from build123d import *

# Parameters (mm, degrees)
SKETCH1_W                    = 94
SKETCH1_H                    = 75
BASE_FLANGE1_DEPTH           = 1.5
EDGE_FLANGE1_DEPTH           = 75
EDGE_FLANGE2_STRIP_W         = 16
EDGE_FLANGE2_STRIP_H         = 1.5
EDGE_FLANGE2_STRIP_CUT_DEPTH = 75
EDGE_FLANGE2_DEPTH           = 75
EDGE_FLANGE3_DEPTH           = 75
EDGE_FLANGE4_STRIP_W         = 16
EDGE_FLANGE4_STRIP_H         = 1.5
EDGE_FLANGE4_STRIP_CUT_DEPTH = 75
EDGE_FLANGE4_DEPTH           = 75
SKETCH18_R                   = 7.5
CUT_EXTRUDE1_DEPTH           = 10
EDGE_FLANGE5_DEPTH           = 94
EDGE_FLANGE6_DEPTH           = 94


# Sheet-metal steps are written as plain solids
with BuildPart() as part:
    # Sketch1 → Base-Flange1 (new body)
    with BuildSketch(Plane.XY):
        Rectangle(SKETCH1_W, SKETCH1_H)
        with BuildLine():
            Line((5, 25.5), (5, 13.5))
            ThreePointArc((5, 13.5), (0, 8.5), (-5, 13.5))
            Line((-5, 13.5), (-5, 25.5))
            ThreePointArc((-5, 25.5), (0, 30.5), (5, 25.5))
        make_face(mode=Mode.SUBTRACT)
        with BuildLine():
            Line((19.583647797, -17.080127019), (9.191342951, -11.080127019))
            ThreePointArc((9.191342951, -11.080127019), (7.361215932, -4.25), (14.191342951, -2.419872981))
            Line((14.191342951, -2.419872981), (24.583647797, -8.419872981))
            ThreePointArc((24.583647797, -8.419872981), (26.413774815, -15.25), (19.583647797, -17.080127019))
        make_face(mode=Mode.SUBTRACT)
        with BuildLine():
            Line((-24.583647797, -8.419872981), (-14.191342951, -2.419872981))
            ThreePointArc((-14.191342951, -2.419872981), (-7.361215932, -4.25), (-9.191342951, -11.080127019))
            Line((-9.191342951, -11.080127019), (-19.583647797, -17.080127019))
            ThreePointArc((-19.583647797, -17.080127019), (-26.413774815, -15.25), (-24.583647797, -8.419872981))
        make_face(mode=Mode.SUBTRACT)
    extrude(amount=-BASE_FLANGE1_DEPTH)

    # Edge-Flange1 section (across the edge) → Edge-Flange1 (add)
    with BuildSketch(Plane(origin=(49, -37.5, 0), x_dir=(-1, 0, 0), z_dir=(0, 1, 0))):
        with BuildLine():
            Line((-1.5, 2), (-1.5, 18.5))
            Line((-1.5, 18.5), (0, 18.5))
            Line((0, 18.5), (0, 2))
            ThreePointArc((0, 2), (0.585786438, 0.585786438), (2, 0))
            Line((2, 0), (2, -1.5))
            ThreePointArc((2, -1.5), (-0.474873734, -0.474873734), (-1.5, 2))
        make_face()
    extrude(amount=EDGE_FLANGE1_DEPTH)

    # Edge-Flange2 strip (across the edge) → Edge-Flange2 strip cut (cut)
    with BuildSketch(Plane(origin=(50.5, 37.5, 18.5), x_dir=(0, 0, -1), z_dir=(0, -1, 0))):
        with Locations((-3, -0.75)):
            Rectangle(EDGE_FLANGE2_STRIP_W, EDGE_FLANGE2_STRIP_H)
    extrude(amount=EDGE_FLANGE2_STRIP_CUT_DEPTH, mode=Mode.SUBTRACT)

    # Edge-Flange2 section (across the edge) → Edge-Flange2 (add)
    with BuildSketch(Plane(origin=(50.5, 37.5, 18.5), x_dir=(0, 0, -1), z_dir=(0, -1, 0))):
        with BuildLine():
            Line((-1.5, 5), (-1.5, 48.5))
            Line((-1.5, 48.5), (0, 48.5))
            Line((0, 48.5), (0, 5))
            ThreePointArc((0, 5), (1.464466094, 1.464466094), (5, 0))
            Line((5, 0), (5, -1.5))
            ThreePointArc((5, -1.5), (0.403805922, 0.403805922), (-1.5, 5))
        make_face()
    extrude(amount=EDGE_FLANGE2_DEPTH)

    # Edge-Flange3 section (across the edge) → Edge-Flange3 (add)
    with BuildSketch(Plane(origin=(-49, 37.5, 0), x_dir=(1, 0, 0), z_dir=(0, -1, 0))):
        with BuildLine():
            Line((-1.5, 2), (-1.5, 18.5))
            Line((-1.5, 18.5), (0, 18.5))
            Line((0, 18.5), (0, 2))
            ThreePointArc((0, 2), (0.585786438, 0.585786438), (2, 0))
            Line((2, 0), (2, -1.5))
            ThreePointArc((2, -1.5), (-0.474873734, -0.474873734), (-1.5, 2))
        make_face()
    extrude(amount=EDGE_FLANGE3_DEPTH)

    # Edge-Flange4 strip (across the edge) → Edge-Flange4 strip cut (cut)
    with BuildSketch(Plane(origin=(-50.5, -37.5, 18.5), x_dir=(0, 0, -1), z_dir=(0, 1, 0))):
        with Locations((-3, -0.75)):
            Rectangle(EDGE_FLANGE4_STRIP_W, EDGE_FLANGE4_STRIP_H)
    extrude(amount=EDGE_FLANGE4_STRIP_CUT_DEPTH, mode=Mode.SUBTRACT)

    # Edge-Flange4 section (across the edge) → Edge-Flange4 (add)
    with BuildSketch(Plane(origin=(-50.5, -37.5, 18.5), x_dir=(0, 0, -1), z_dir=(0, 1, 0))):
        with BuildLine():
            Line((-1.5, 5), (-1.5, 48.5))
            Line((-1.5, 48.5), (0, 48.5))
            Line((0, 48.5), (0, 5))
            ThreePointArc((0, 5), (1.464466094, 1.464466094), (5, 0))
            Line((5, 0), (5, -1.5))
            ThreePointArc((5, -1.5), (0.403805922, 0.403805922), (-1.5, 5))
        make_face()
    extrude(amount=EDGE_FLANGE4_DEPTH)

    # Sketch18 → Cut-Extrude1 (cut)
    with BuildSketch(Plane.XY.offset(20)):
        with Locations((70, 17.5)):
            Circle(SKETCH18_R)
        with Locations(Location((-70, 17.5, 0), (0, 0, 180))):
            Circle(SKETCH18_R)
    extrude(amount=-CUT_EXTRUDE1_DEPTH, mode=Mode.SUBTRACT)

    # Edge-Flange5 section (across the edge) → Edge-Flange5 (add)
    with BuildSketch(Plane(origin=(-47, 37.925276208, -1.5), x_dir=(0, -0.8660254037844364, -0.5000000000000041), z_dir=(1, 0, 0))):
        with BuildLine():
            Line((-1.5, 0.425276208), (-1.5, 20))
            Line((-1.5, 20), (0, 20))
            Line((0, 20), (0, 0.425276208))
            ThreePointArc((0, 0.425276208), (0.098685688, 0.056976208), (0.3683, -0.212638104))
            Line((0.3683, -0.212638104), (-0.3817, -1.51167621))
            ThreePointArc((-0.3817, -1.51167621), (-1.200352418, -0.693023792), (-1.5, 0.425276208))
        make_face()
    extrude(amount=EDGE_FLANGE5_DEPTH)

    # Edge-Flange6 section (across the edge) → Edge-Flange6 (add)
    with BuildSketch(Plane(origin=(47, -37.925276208, -1.5), x_dir=(0, 0.8660254037844364, -0.5000000000000041), z_dir=(-1, 0, 0))):
        with BuildLine():
            Line((-1.5, 0.425276208), (-1.5, 20))
            Line((-1.5, 20), (0, 20))
            Line((0, 20), (0, 0.425276208))
            ThreePointArc((0, 0.425276208), (0.098685688, 0.056976208), (0.3683, -0.212638104))
            Line((0.3683, -0.212638104), (-0.3817, -1.51167621))
            ThreePointArc((-0.3817, -1.51167621), (-1.200352418, -0.693023792), (-1.5, 0.425276208))
        make_face()
    extrude(amount=EDGE_FLANGE6_DEPTH)


solid = part.part
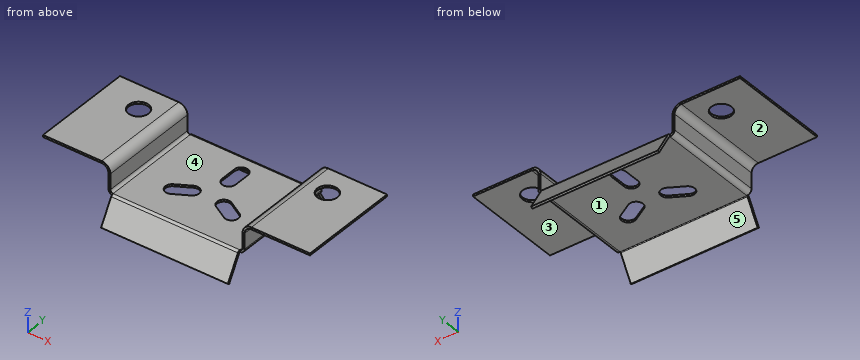
Model file for the job. Use its own axes, mm. Face numbers are marked on the shaded views. A direction names the side the tool comes from. Give positions to 0.01 mm unless a question says otherwise; leave off trailing zeros. Loops run counter-clockwise (first coordinate to the right, second up) from the corner with the lowest first, then second, coordinate; pieces in that order, holes last. Notation, with made-up numbers: (-1, -23.5) -> (45, -23.5) arc R15 cw to (45, -14.5) -> close; hole circle Ø5 at (-26.75, 27.25). An arc over 180 degrees is marked (long way). Use a Markdown table: item, result. Add a question column.
(1) Drop flat-ended pins along their axis: pin 1 Ø9 at (y, z) = (-16, 5) entering from -X; pin 2 Ø13 at (y, z) = (44.5, -10.5) entering from -X; pin 3 Ø10 at (y, z) = (12.5, 12.5) entering from +X. Give the stop position or say it passes through.
(2) Slice it at A-A on y = 17.5. Give the number of separate pieces and of enclosed holes in the cut face, and give its area (3 significant figures).
(3) Slice it at B-B on z = 4. List the corners of the cut face in (x, y).
(4) Slice it at C-C on x = 0. List the corners of the cut face in (y, z), and give its area (3 significant figures).
(5) Slice it at D-D on x = 29.5. List the corners of the cut face in (y, z).
(6) Mould opens along X. For the marked faces 4 and 5 say: +X half, -X half, draft (parallel to the pull), parting line (faces both ways), or undercut.
(7) Wall check: line 1 along Y through (x, z) = (-70, 19.2); line 2 along X through (y, z) = (17, 19); line 3 along Z through (x, y) = (0.5, -30). Give the ranges that are in metal, low to high.
(8) Tool access for the marked faces 1, 2 and 3: list every direction of +Z, -Z, +X, -X, +Y, -Y with a clear straight run to the whole face (end or side of a thin tool).
Filled sheet:
| question | item | result |
|---|---|---|
| 1 | pin 1 | x = -50.5 |
| 1 | pin 2 | x = -47 |
| 1 | pin 3 | x = 52.5 |
| 2 | separate pieces | 4 |
| 2 | enclosed holes | 0 |
| 2 | area | 286 mm2 |
| 3 | outline | (-50.5, -37.5) -> (-49, -37.5) -> (-49, 37.5) -> (-50.5, 37.5) -> close; (49, -37.5) -> (50.5, -37.5) -> (50.5, 37.5) -> (49, 37.5) -> close |
| 4 | outline | (-49.22, -18.07) -> (-47.93, -18.82) -> (-38.14, -1.87) arc R0.74 cw to (-37.5, -1.5) -> (8.5, -1.5) -> (8.5, 0) -> (-37.5, 0) arc R2.24 ccw to (-39.44, -1.12) -> close; (30.5, -1.5) -> (37.5, -1.5) arc R0.74 cw to (38.14, -1.87) -> (47.93, -18.82) -> (49.22, -18.07) -> (39.44, -1.12) arc R2.24 ccw to (37.5, 0) -> (30.5, 0) -> close |
| 4 | area | 143 mm2 |
| 5 | outline | (-49.22, -18.07) -> (-47.93, -18.82) -> (-38.14, -1.87) arc R0.74 cw to (-37.5, -1.5) -> (37.5, -1.5) arc R0.74 cw to (38.14, -1.87) -> (47.93, -18.82) -> (49.22, -18.07) -> (39.44, -1.12) arc R2.24 ccw to (37.5, 0) -> (-37.5, 0) arc R2.24 ccw to (-39.44, -1.12) -> close |
| 6 | face 4 | undercut |
| 6 | face 5 | draft |
| 7 | line 1 | -37.5 to 10, 25 to 37.5 |
| 7 | line 2 | -99 to -77.48, -62.52 to -52.04, 52.04 to 62.52, 77.48 to 99 |
| 7 | line 3 | -1.5 to 0 |
| 8 | face 1 | -Z, +X, -X |
| 8 | face 2 | -Z, -X, +Y, -Y |
| 8 | face 3 | -Z, +X, +Y, -Y |
